Part model, mm, in its own coordinate system. A direction names the side the tool comes from. Round coordinates to 2 decimals unless told otherwise and drop trailing zeros. Loops run counter-clockwise (first coordinate to the right, second up) from the corner with the lowest first, then second, coordinate; pieces in that order, holes last.
1) Band-saw the part on D-D, the plane y = 22. Write the cut outline in (x, z).
2) 3-axis set-ups, long thin cutter, end or side, ignore diameter. For faces 4 (the flat face through (15, 35, 30)), 5 (the flat face through (-19, 10, 2)), 6 (the flat face through (11, 19, 20)), 7 (the flat face through (5, 20, 0)), 8 (the flat face through (-18, 25, 10)): which of +Z, -Z, +X, -X, +Y, -Y reach the whole face in a straight line?
3) Band-saw the part on A-A, the plane y = 11. Write the cut outline in (x, z).
4) Drop flat-ended pins along their axis: P1, Ø9, axis at x = -21.5, y = 28, coming from the +Z side; P2, Ø1.5, axis at x = 11, y = 24.5, coming from the +Z side; P3, Ø3, axis at y = 14.5, z = 15.5, coming from the -X side. Give the stop position or say it passes through.
5) Mould opens along Y. For faces 1 (the cylindrical face through (17.307, 10.564, 9.86)), 2 (the flat face through (-25, 25, -10)), 3 (the flat face through (15, 30, 25)) say: +Y half, -Y half, draft (parallel to the pull), parting line (faces both ways), or undercut.
6) Probe line 1 (Y direction, x = -10, z = 2.5); line 2 (Z direction, x = -24, y = 25); line 3 (Z direction, x = 23, y = 14). List the from-to ranges inside material, lowest first.
7) Band-saw the part on B-B, the plane x = 15. Write the cut outline in (y, z).
8) Band-saw the part on C-C, the plane z = 8. Write the cut outline in (x, y).
from build123d import *

# Parameters (mm, degrees)
F0_W     = 30
F0_H     = 40
F0_R     = 5
F1_DEPTH = 20
F2_W     = 30
F2_H     = 10
F3_DEPTH = 10
F4_W     = 30
F4_H     = 10
F5_DEPTH = 30
F6_R     = 5
F7_DEPTH = 25
F8_W     = 10
F8_H     = 30
F9_DEPTH = 10


with BuildPart() as f1:
    # F0 (on Top) → F1 (new body)
    with BuildSketch(Plane.XY):
        with Locations((15, 20)):
            Rectangle(F0_W, F0_H)
        with Locations((15, 15)):
            Circle(F0_R, mode=Mode.SUBTRACT)
    extrude(amount=F1_DEPTH)

    # F2 (on face) → F3 (join)
    with BuildSketch(Plane.XY.offset(20)):
        with Locations((15, 35)):
            Rectangle(F2_W, F2_H)
    extrude(amount=F3_DEPTH)

    # F4 (on face) → F5 (join)
    with BuildSketch(Plane(origin=(0, 0, 0), x_dir=(0, -1, 0), z_dir=(-1, 0, 0))):
        with Locations((-25, 5)):
            Rectangle(F4_W, F4_H)
    extrude(amount=F5_DEPTH)

    # F6 (on face) → F7 (cut)
    with BuildSketch(Plane.XY.offset(10)):
        with Locations((-10, 25)):
            Circle(F6_R)
    extrude(amount=-F7_DEPTH, mode=Mode.SUBTRACT)

    # F8 (on face) → F9 (join)
    with BuildSketch(Plane(origin=(0, 0, 0), x_dir=(1, 0, 0), z_dir=(0, 0, -1))):
        with Locations((-25, -25)):
            Rectangle(F8_W, F8_H)
    extrude(amount=F9_DEPTH)


solid = f1.part
Reported:
1. outline: (-30, -10) - (-20, -10) - (-20, 0) - (-14, 0) - (-14, 10) - (-30, 10) - close; (-6, 0) - (30, 0) - (30, 20) - (0, 20) - (0, 10) - (-6, 10) - close
2. face 4: +Z, +X, -X, +Y, -Y
2. face 5: +Z, -Z, -X, -Y
2. face 6: +Z, +X, -X, -Y
2. face 7: -Z, +X, +Y, -Y
2. face 8: +Z, -X, +Y, -Y
3. outline: (-30, -10) - (-20, -10) - (-20, 0) - (12, 0) - (12, 20) - (0, 20) - (0, 10) - (-30, 10) - close; (18, 0) - (30, 0) - (30, 20) - (18, 20) - close
4. P1: stops at z = 10
4. P2: stops at z = 20
4. P3: stops at x = 0
5. face 1: undercut
5. face 2: draft
5. face 3: -Y half
6. line 1: y = 10 to 20, 30 to 40
6. line 2: z = -10 to 10
6. line 3: z = 0 to 20
7. outline: (0, 0) - (10, 0) - (10, 20) - (0, 20) - close; (20, 0) - (40, 0) - (40, 30) - (30, 30) - (30, 20) - (20, 20) - close
8. outline: (-30, 10) - (0, 10) - (0, 0) - (30, 0) - (30, 40) - (-30, 40) - close; hole circle Ø10 at (-10, 25); hole circle Ø10 at (15, 15)
